Work out the finished part from the listing and answer in its coordinate system (mm). Face numbers are marked on the shaded views. A direction names the side the tool comes from. Give positions to 0.01 mm unless a question says otherwise; leave off trailing zeros. Write each loop counter-clockwise with the first axis right and the second up, starting at its lowest first coordinate (ties: lowest second). Pieces come first, ordered by that corner, then holes. Notation, with made-up numbers: (82, -10) -> (117, -10) arc R25 ccw to (117, 11) -> close; hole circle Ø10 at (8.25, -25.75). An arc over 180 degrees is marked (long way). Use a Markdown table: item, result. Add a question column.
Q1. Section C-C, the plane y = 2 is taken. Give the vertices of the cut face in (x, z), plus the area to 3 significant figures.
Q2. Each of these flat-tipped pins is pushed along its axis until it touches: pin 1 Ø1.5 at (x, z) = (81, 4.5) entering from -Y; pin 2 Ø5 at (y, z) = (18, 5) entering from +X; pin 3 Ø0.9 at (x, z) = (81, 3.5) entering from +Y. Where does it stop, or does it pass through?
Q3. For a pull along Y with two mould halves and no side action, classify the marked faces 4, 5 and 6 as pulls with the +Y half, pulls with the -Y half, needs draft (parallel to the pull), parting line crosses it, or undercut.
Q4. Section B-B, the plane z = 8.5 is taken. Give the vertices of the cut face in (x, y).
Q5. Section D-D, the plane y = 21.5 is taken. Give the vertices of the cut face in (x, z), plus the area to 3 significant figures.
Q6. Section A-A, the plane x = 44.5 is taken. Give the vertices of the cut face in (y, z).
Q7. For the marked faces 1, 2 and 3, determine the directions among +Z, -Z, +X, -X, +Y, -Y from which every point of the face is accessible in a straight line to the end or side of a thin tool.
Q8. Consider line 1 (Y direction, x = 64, z = 5.75); line 2 (Y direction, x = 2.5, z = 6.5); line 3 (X direction, y = 10.5, z = 7.5). Determine where each line is inside the solid, lowest interval first.
from build123d import *

# Parameters (mm, degrees)
ESQUISSE1_W             = 85.5
ESQUISSE1_H             = 34.5
ESQUISSE1_W_2           = 80.5
ESQUISSE1_H_2           = 29.5
BOSS_EXTRU_1_DEPTH      = 10
CONG_1_R                = 6
CONG_2_R                = 6
ESQUISSE3_W             = 10
ESQUISSE3_H             = 22.5
ENL_V_MAT_EXTRU_1_DEPTH = 10


with BuildPart() as part:
    # Esquisse1 → Boss.-Extru.1 (new body)
    with BuildSketch(Plane.XY):
        with Locations((40.25, 14.75)):
            Rectangle(ESQUISSE1_W, ESQUISSE1_H)
        with Locations((40.25, 14.75)):
            Rectangle(ESQUISSE1_W_2, ESQUISSE1_H_2, mode=Mode.SUBTRACT)
    extrude(amount=BOSS_EXTRU_1_DEPTH)

    # Congé1
    cong_1_edges = [part.edges().sort_by_distance(p)[0] for p in [
        (0, 29.5, 5),
        (0, 0, 5),
        (80.5, 0, 5),
        (80.5, 29.5, 5),
    ]]
    fillet(cong_1_edges, radius=CONG_1_R)

    # Congé2
    cong_2_edges = [part.edges().sort_by_distance(p)[0] for p in [
        (-2.5, 32, 5),
        (83, 32, 5),
        (83, -2.5, 5),
        (-2.5, -2.5, 5),
    ]]
    fillet(cong_2_edges, radius=CONG_2_R)

    # Esquisse3 → Enlèv. mat.-Extru.1 (cut)
    with BuildSketch(Plane(origin=(83, 0, 0), x_dir=(0, 0, -1), z_dir=(1, 0, 0))):
        with Locations((-5, 14.75)):
            Rectangle(ESQUISSE3_W, ESQUISSE3_H)
    extrude(amount=-ENL_V_MAT_EXTRU_1_DEPTH, mode=Mode.SUBTRACT)


solid = part.part
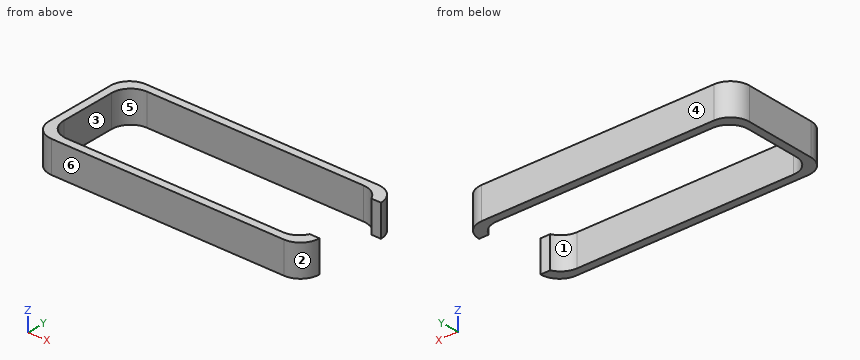
Result set:
| question | item | result |
|---|---|---|
| 1 | outline | (-2.31, 0) -> (1.53, 0) -> (1.53, 10) -> (-2.31, 10) -> close; (78.97, 0) -> (82.81, 0) -> (82.81, 10) -> (78.97, 10) -> close |
| 1 | area | 76.7 mm2 |
| 2 | pin 1 | stops at y = -1.54 |
| 2 | pin 2 | stops at x = 0 |
| 2 | pin 3 | stops at y = 30.84 |
| 3 | face 4 | pulls with the +Y half |
| 3 | face 5 | undercut |
| 3 | face 6 | pulls with the -Y half |
| 4 | outline | (-2.5, 3.5) arc R6 ccw to (3.5, -2.5) -> (77, -2.5) arc R6 ccw to (83, 3.5) -> (79.95, 3.5) arc R6 cw to (74.5, 0) -> (6, 0) arc R6 cw to (0, 6) -> (0, 23.5) arc R6 cw to (6, 29.5) -> (74.5, 29.5) arc R6 cw to (79.95, 26) -> (83, 26) arc R6 ccw to (77, 32) -> (3.5, 32) arc R6 ccw to (-2.5, 26) -> close |
| 5 | outline | (-2.5, 0) -> (0, 0) -> (0, 10) -> (-2.5, 10) -> close |
| 5 | area | 25.0 mm2 |
| 6 | outline | (-2.5, 0) -> (0, 0) -> (0, 10) -> (-2.5, 10) -> close; (29.5, 0) -> (32, 0) -> (32, 10) -> (29.5, 10) -> close |
| 7 | face 1 | +Z, -Z |
| 7 | face 2 | +Z, -Z, +X, -Y |
| 7 | face 3 | +Z, -Z, +X |
| 8 | line 1 | y = -2.5 to 0, 29.5 to 32 |
| 8 | line 2 | y = -2.42 to 1.13, 28.37 to 31.92 |
| 8 | line 3 | x = -2.5 to 0 |
